Read the model definition and answer for the solid it produces. Units are mm, in the model's axes. Round coordinates to 2 decimals unless told otherwise and drop trailing zeros. Order: outer loops, then holes, each group sorted by start corner. A loop starts at its lowest first (then second) coordinate and runs counter-clockwise, first axis right, second up. Notation, with made-up numbers: (36.5, 75.5) -> (92.5, 75.5) arc R22 cw to (92.5, 107.5) -> close; hole circle Ø5 at (8, 82). An arc over 180 degrees is marked (long way). Use a Markdown table: item, result. Add a question column.
1. Consider L1, parallel to Y at x = -37, z = -33; L2, parallel to X at y = 10.25, z = -23.5; L3, parallel to X at y = 10.75, z = -34. Determine where each line is inside the solid, lowest interval first. Write a range as [from, to].
2. Section C-C, the plane z = -39 is taken. Give the vertices of the cut face in (x, y), then the cut area to 3 significant figures.
3. Section B-B, the plane y = 10 is taken. Give the vertices of the cut face in (x, z) (1 decimal), then the cut area to 3 significant figures.
4. The mould has two halves that part along Y. Classify faces 1 (the face through (-4.831, 11.597, -30.961)), 2 (the face through (-5, 8, -21.2)), 3 (the face through (-36.169, 8.403, -30.961)), 4 (the face through (-21, 2, -33)): +Y half, -Y half, draft (parallel to the pull), parting line (faces both ways), or undercut.
5. Given pin 1 (6 mm diameter, centred on x = -25.5, y = 9, fed in from +Z), flat-ended and moving along its own axis, determine where the tip first touches the part or whether it passes through.
6. Section A-A, the plane x = -37 is taken. Give the vertices of the cut face in (y, z).
Autodesk Inventor part; units mm, degrees
ref_plane "Work Plane1" through (-20.5, 0, -41) normal (1, 0, 0) x (0, 0, -1)
ref_plane "YZ Plane" through (0, 0, 0) normal (1, 0, 0) x (0, 1, 0)
ref_plane "XZ Plane" through (0, 0, 0) normal (0, 1, 0) x (-1, 0, 0)
sketch "Sketch1" plane through (0, 0, 0) normal (0, 1, 0) x (-1, 0, 0)
  line L0 (0, 0) -> (41, 0)
  line L1 (41, 0) -> (41, -41)
  line L2 (41, -41) -> (0, -41)
  line L3 (0, -41) -> (0, 0)
  dimension "d0" = 41
  dimension "d1" = 41
extrude "Extrusion1" add sketch "Sketch1" along normal blind 9.5
sketch "Sketch3" plane through (0, 9.5, 0) normal (0, 1, 0) x (1, 0, 0)
  circle A0 centre (-20.5, 20.5) radius 10
  point P0 (0, 0)
  dimension "d5" = 20
extrude "Extrusion2" cut sketch "Sketch3" against normal blind 10
sketch "Sketch4" plane through (0, 9.5, 0) normal (0, 1, 0) x (1, 0, 0)
  circle A0 centre (-20.5, 20.5) radius 10
  circle A1 centre (-20.5, 20.5) radius 11.75
  point P0 (0, 0)
  dimension "d8" = 23.5
extrude "Extrusion3" cut sketch "Sketch4" against normal blind 5
sketch "Sketch5" plane through (0, 9.5, 0) normal (0, 1, 0) x (1, 0, 0)
  line L0 (-41, 41) -> (-41, 0)
  line L1 (-41, 0) -> (0, 0)
  line L2 (0, 0) -> (0, 41)
  line L3 (0, 41) -> (-41, 41)
  line L4 (-41, 41) -> (-41, 0)
  circle A0 centre (-20.5, 20.5) radius 11.75
  circle A1 centre (-20.5, 20.5) radius 10
extrude "Extrusion4" add sketch "Sketch5" along normal blind 4.5 contours L3 L2 L1 L0 | A0
sketch "Sketch6" plane through (-41, 0, 0) normal (0, 0, 1) x (1, 0, 0)
  line L0 (0, 0) -> (0, 14)
  line L1 (0, 14) -> (41, 14)
  line L2 (41, 14) -> (41, 0)
  line L3 (41, 0) -> (0, 0)
  line L4 (0, 0) -> (0, 14)
extrude "Extrusion5" cut sketch "Sketch6" against normal blind 20.5
sketch "Sketch8" plane through (-41, 0, -20.5) normal (0, 0, 1) x (1, 0, 0)
  circle A0 centre (4, 10) radius 1.8
  point P0 (41, 0)
  dimension "d15" = 3.6
extrude "Extrusion6" cut sketch "Sketch8" against normal blind 20.5
ref_plane "Work Plane1" through (-20.5, 0, -41) normal (1, 0, 0) x (0, 0, -1)
mirror "Mirror1" about plane through (-20.5, 0, -41) normal (1, 0, 0) of "Extrusion6"
sketch "Sketch9" plane through (-41, 0, -20.5) normal (0, 0, 1) x (1, 0, 0)
  line L0 (10.5, 14) -> (10.5, 9.5)
  line L1 (8.75, 4.5) -> (10.5, 4.5)
  line L2 (10.5, 9.5) -> (8.75, 9.5)
  line L3 (8.75, 9.5) -> (8.75, 4.5)
  line L4 (8.75, 4.5) -> (10.5, 4.5)
  line L5 (10.5, 4.5) -> (10.5, 9.5)
  point P0 (41, 0)
sketch "Sketch11" plane through (0, 4.5, 0) normal (0, 1, 0) x (1, 0, 0)
  arc A0 (-10.5, 20.5) -> (-30.5, 20.5) centre (-20.5, 20.5) ccw
  arc A1 (-9.625, 20.5) -> (-31.375, 20.5) centre (-20.5, 20.5) ccw
  line L0 (-41, 41) -> (-41, 20.5)
  point P0 (0, 0)
sweep "Sweep1" add profiles "Sketch9" path "Sketch11" path curves A1
sketch "Sketch12" plane through (-41, 0, -20.5) normal (0, 0, 1) x (1, 0, 0)
  line L0 (10.5, 14) -> (10.5, 0)
  circle A0 centre (10.5, 7) radius 1.6
  point P0 (41, 0)
  dimension "d21" = 3.2
sketch3d "3D Sketch1"
  arc A0 (-30.5, 14, -20.5) -> (-27.5711, 14, -27.5711) centre (-20.5, 14, -20.5) ccw
  arc A1 (-27.5711, 14, -27.5711) -> (-20.5, 14, -30.5) centre (-20.5, 14, -20.5) ccw
  arc A2 (-20.5, 14, -30.5) -> (-13.4289, 14, -27.5711) centre (-20.5, 14, -20.5) ccw
  arc A3 (-13.4289, 14, -27.5711) -> (-10.5, 14, -20.5) centre (-20.5, 14, -20.5) ccw
sweep "Sweep2" cut profiles "Sketch12" path "3D Sketch1"
sketch "Sketch13" plane through (0, 0, 0) normal (0, -1, 0) x (1, 0, 0)
  line L0 (-53.975, -9.525) -> (46.0375, -9.525)
  line L1 (46.0375, -9.525) -> (46.0375, -71.4375)
  line L2 (46.0375, -71.4375) -> (-53.975, -71.4375)
  line L3 (-53.975, -71.4375) -> (-53.975, -9.525)
  point P0 (0, 0)
extrude "Extrusion7" cut sketch "Sketch13" against normal blind 2
sketch "Sketch14" plane through (-41, 0, -20.5) normal (0, 0, 1) x (1, 0, 0)
  line L0 (-1.5875, 15.875) -> (46.0375, 15.875)
  line L1 (46.0375, 15.875) -> (46.0375, -1.5875)
  line L2 (46.0375, -1.5875) -> (-1.5875, -1.5875)
  line L3 (-1.5875, -1.5875) -> (-1.5875, 15.875)
  point P0 (41, 0)
extrude "Extrusion8" cut sketch "Sketch14" against normal blind 0.7
sketch "Sketch15" plane through (0, 14, 0) normal (0, 1, 0) x (1, 0, 0)
  arc A0 (-10.5245, 21.2) -> (-30.4755, 21.2) centre (-20.5, 20.5) ccw
  circle A1 centre (-20.5, 20.5) radius 10.9575
  point P0 (0, 0)
  dimension "d28" = 21.915
extrude "Extrusion9" cut sketch "Sketch15" against normal blind 15
sketch "Sketch18" plane through (-41, 0, -21.2) normal (0, 0, 1) x (1, 0, 0)
  point P0 (41, 0)
sketch "Sketch19" plane through (-41, 0, -21.2) normal (0, 0, 1) x (1, 0, 0)
  circle A0 centre (9.5649, 7) radius 1.6
  point P0 (41, 0)
  dimension "d34" = 3.2
sketch "Sketch20" plane through (0, 14, 0) normal (0, 1, 0) x (1, 0, 0)
  arc A0 (-9.5649, 21.2) -> (-31.4351, 21.2) centre (-20.5, 20.5) ccw
  circle A1 centre (-20.5, 20.5) radius 10.9575
  point P0 (0, 0)
sweep "Sweep4" cut profiles "Sketch19" path "Sketch20" path curves A1
properties part number "8.1 peristaltic pump lid 3mm"
Verdict:
| question | item | result |
|---|---|---|
| 1 | L1 | y = [2, 8.2], [11.8, 14] |
| 1 | L2 | x = [-41, -38.78], [-35.22, -31.04], [-9.96, -5.78], [-2.22, 0] |
| 1 | L3 | x = [-41, -38.64], [-35.36, -5.64], [-2.36, 0] |
| 2 | outline | (-41, 2) -> (0, 2) -> (0, 14) -> (-41, 14) -> close; hole circle Ø3.6 at (-37, 10); hole circle Ø3.6 at (-4, 10) |
| 2 | area | 472 mm2 |
| 3 | outline | (-41, -41) -> (-38.8, -41) -> (-38.8, -21.2) -> (-41, -21.2) -> close; (-35.2, -41) -> (-5.8, -41) -> (-5.8, -21.2) -> (-9.6, -21.2) arc R11 cw to (-31.4, -21.2) -> (-35.2, -21.2) -> close; (-2.2, -41) -> (0, -41) -> (0, -21.2) -> (-2.2, -21.2) -> close |
| 3 | area | 496 mm2 |
| 4 | face 1 | undercut |
| 4 | face 2 | draft |
| 4 | face 3 | undercut |
| 4 | face 4 | -Y half |
| 5 | pin 1 | stops at z = -27.99 |
| 6 | outline | (2, -41) -> (8.2, -41) -> (8.2, -21.2) -> (2, -21.2) -> close; (11.8, -41) -> (14, -41) -> (14, -21.2) -> (11.8, -21.2) -> close |
